Geometry check sheet. Reference: the model listing, model coordinates, mm. Face numbers are marked on the shaded views. Give positions to 0.01 mm unless a question says otherwise; leave off trailing zeros. Order: outer loops, then holes, each group sorted by start corner. A loop starts at its lowest first (then second) coordinate and runs counter-clockwise, first axis right, second up.
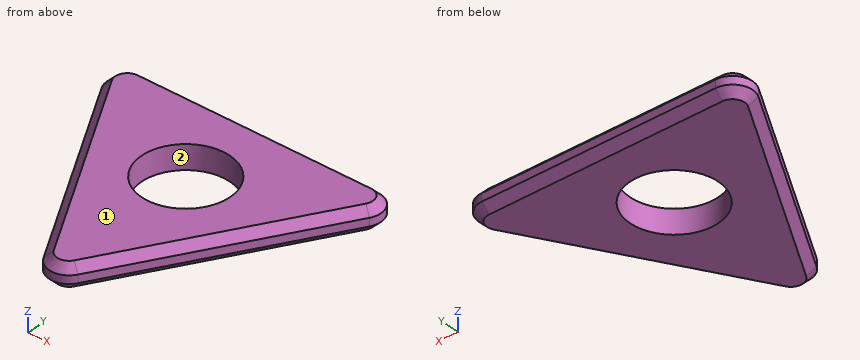
```python
from build123d import *

# Parameters (mm, degrees)
F0_R     = 11
F1_DEPTH = 6
F2_SIZE  = 2


# Not quite as in the source:
# - a feature of the source that left no trace in its solid (it failed there, or was rolled back) is left out


with BuildPart() as f1:
    # F0 (on Top) → F1 (new body)
    with BuildSketch(Plane.XY):
        with BuildLine():
            Line((29.4397459622, 21.9970452561), (-29.4397459622, 21.9970452561))
            ThreePointArc((-29.4397459622, 21.9970452561), (-33.7698729811, 19.4970452561), (-33.7698729811, 14.4970452561))
            Line((-33.7698729811, 14.4970452561), (-4.3301270189, -36.4940905122))
            ThreePointArc((-4.3301270189, -36.4940905122), (0, -38.9940905122), (4.3301270189, -36.4940905122))
            Line((4.3301270189, -36.4940905122), (33.7698729811, 14.4970452561))
            ThreePointArc((33.7698729811, 14.4970452561), (33.7698729811, 19.4970452561), (29.4397459622, 21.9970452561))
        make_face()
        Circle(F0_R, mode=Mode.SUBTRACT)
    extrude(amount=F1_DEPTH)

    # F2
    f2_edges = [f1.edges().sort_by_distance(p)[0] for p in [
        (-19.05, -10.998523, 6),
        (-19.05, -10.998523, 0),
        (0, 21.997045, 6),
        (33.769873, 19.497045, 0),
        (33.769873, 19.497045, 6),
        (0, 21.997045, 0),
        (-33.769873, 19.497045, 0),
        (-33.769873, 19.497045, 6),
        (0, -38.994091, 0),
        (0, -38.994091, 6),
        (19.05, -10.998523, 0),
        (19.05, -10.998523, 6),
    ]]
    chamfer(f2_edges, length=F2_SIZE)


solid = f1.part
```
Q1. Thickness scan on L1, parallel to X at y = -2, z = 5.45; L2, parallel to X at y = -1, z = 0.75; L3, parallel to Y at x = -7, z = 4.8. Record the ranges inside material, lowest first.
Q2. Cross-section at C-C, the plane z = 5. Record the boundary of the cut face in (x, y), and give its area (3 significant figures).
Q3. Gauge pin test, flat ends, axial feed: P1, Ø1.5, axis at x = -23.5, y = -5, coming from the -Z side; P2, Ø1.5, axis at x = 10.5, z = 3.5, coming from the -Y side; P3, Ø1.5, axis at y = -13, z = 5, coming from the -X side; P4, Ø1, axis at y = -19, z = 2, coming from the -X side. Record the tip position at first contact, or that the pin passes through.
Q4. Release check for a two-part mould opening along Y. For the marked faces 1 and 2 record: pulls with the +Y half, pulls with the -Y half, needs draft (parallel to the pull), parting line crosses it, or undercut.
Q5. Cross-section at D-D, the plane x = -17.5. Record the boundary of the cut face in (y, z), and give its area (3 significant figures).
Q6. Cross-section at A-A, the plane y = 4. Record the boundary of the cut face in (x, z).
Q7. Cross-section at B-B, the plane x = 0. Record the boundary of the cut face in (y, z), and give its area (3 significant figures).
Answers follow:
1. L1: x = -22.57 to -10.82, 10.82 to 22.57
1. L2: x = -23.38 to -10.95, 10.95 to 23.38
1. L3: y = -30.27 to -8.49, 8.49 to 21.2
2. outline: (-32.9, 15) - (-3.46, -35.99) arc R4 ccw to (3.46, -35.99) - (32.9, 15) arc R4 ccw to (29.44, 21) - (-29.44, 21) arc R4 ccw to start; hole circle Ø22 at (0, 0)
2. area: 1,880 mm2
3. P1: passes through
3. P2: stops at y = -27.11
3. P3: stops at x = -17.71
3. P4: stops at x = -14.72
4. face 1: needs draft
4. face 2: undercut
5. outline: (-13.68, 2) - (-9.68, 0) - (20, 0) - (22, 2) - (22, 4) - (20, 6) - (-9.68, 6) - (-13.68, 4) - close
5. area: 202 mm2
6. outline: (-27.71, 2) - (-25.4, 0) - (-10.25, 0) - (-10.25, 6) - (-25.4, 6) - (-27.71, 4) - close; (10.25, 0) - (25.4, 0) - (27.71, 2) - (27.71, 4) - (25.4, 6) - (10.25, 6) - close
7. outline: (-38.99, 2) - (-36.99, 0) - (-11, 0) - (-11, 6) - (-36.99, 6) - (-38.99, 4) - close; (11, 0) - (20, 0) - (22, 2) - (22, 4) - (20, 6) - (11, 6) - close
7. area: 226 mm2
